```python
from build123d import *

# Parameters (mm, degrees)
ESQUISSE1_R             = 1.66
BOSS_EXTRU_1_DEPTH      = 2.5
ESQUISSE2_W             = 13.135596865
ESQUISSE2_H             = 97.305440857
ENL_V_MAT_EXTRU_1_DEPTH = 3.5


with BuildPart() as part:
    # Esquisse1 → Boss.-Extru.1 (new body)
    with BuildSketch(Plane.XY):
        with BuildLine():
            Line((-29.728572008, 42.160761401), (-21.428572008, 42.160761401))
            Line((-21.428572008, 42.160761401), (21.971427992, 42.160761401))
            Line((21.971427992, 42.160761401), (30.271427992, 42.160761401))
            Line((30.271427992, 42.160761401), (30.271427992, 36.160761401))
            ThreePointArc((30.271427992, 36.160761401), (25.904827727, 32.472835586), (24.271427992, 26.995610011))
            Line((24.271427992, 26.995610011), (24.271427992, -25.67408721))
            ThreePointArc((24.271427992, -25.67408721), (25.904827727, -31.151312785), (30.271427992, -34.839238599))
            Line((30.271427992, -34.839238599), (30.271427992, -40.839238599))
            Line((30.271427992, -40.839238599), (21.971427992, -40.839238599))
            Line((21.971427992, -40.839238599), (-21.428572008, -40.839238599))
            Line((-21.428572008, -40.839238599), (-29.728572008, -40.839238599))
            Line((-29.728572008, -40.839238599), (-29.728572008, -34.839238599))
            ThreePointArc((-29.728572008, -34.839238599), (-25.361971742, -31.151312785), (-23.728572008, -25.67408721))
            Line((-23.728572008, -25.67408721), (-23.728572008, 26.995610011))
            ThreePointArc((-23.728572008, 26.995610011), (-25.361971742, 32.472835586), (-29.728572008, 36.160761401))
            Line((-29.728572008, 36.160761401), (-29.728572008, 42.160761401))
        make_face()
        with Locations((-25.578572008, 39.160761401)):
            Circle(ESQUISSE1_R, mode=Mode.SUBTRACT)
        with Locations((26.121427992, 39.160761401)):
            Circle(ESQUISSE1_R, mode=Mode.SUBTRACT)
        with Locations((-25.578572008, -37.839238599)):
            Circle(ESQUISSE1_R, mode=Mode.SUBTRACT)
        with Locations((26.121427992, -37.839238599)):
            Circle(ESQUISSE1_R, mode=Mode.SUBTRACT)
        with BuildLine():
            Line((-9.728572008, 30.929161254), (10.271427992, 30.929161254))
            ThreePointArc((10.271427992, 30.929161254), (13.806961898, 29.46469516), (15.271427992, 25.929161254))
            Line((15.271427992, 25.929161254), (15.271427992, -24.607638453))
            ThreePointArc((15.271427992, -24.607638453), (13.806961898, -28.143172359), (10.271427992, -29.607638453))
            Line((10.271427992, -29.607638453), (-9.728572008, -29.607638453))
            ThreePointArc((-9.728572008, -29.607638453), (-13.264105914, -28.143172359), (-14.728572008, -24.607638453))
            Line((-14.728572008, -24.607638453), (-14.728572008, 25.929161254))
            ThreePointArc((-14.728572008, 25.929161254), (-13.264105914, 29.46469516), (-9.728572008, 30.929161254))
        make_face(mode=Mode.SUBTRACT)
    extrude(amount=BOSS_EXTRU_1_DEPTH)

    # Esquisse2 → Enlèv. mat.-Extru.1 (cut, through all)
    with BuildSketch(Plane(origin=(0, 0, 0), x_dir=(-1, 0, 0), z_dir=(0, 0, -1))):
        with Locations((-35.339226425, 0.262800476)):
            Rectangle(ESQUISSE2_W, ESQUISSE2_H)
        with Locations((34.79637044, 0.262800476)):
            Rectangle(ESQUISSE2_W, ESQUISSE2_H)
    extrude(amount=-ENL_V_MAT_EXTRU_1_DEPTH, mode=Mode.SUBTRACT)


solid = part.part
```
Work out the finished part from the listing and answer in its coordinate system (mm). A direction names the side the tool comes from. Give positions to 0.01 mm unless a question says otherwise; leave off trailing zeros. Loops run counter-clockwise (first coordinate to the right, second up) from the corner with the lowest first, then second, coordinate; pieces in that order, holes last. Notation, with made-up numbers: (50, -20) -> (77, -20) arc R13 cw to (77, 0) -> close; hole circle Ø6 at (16.25, 33). An arc over 180 degrees is marked (long way). Write item = value, one per line. Start each with the question number.
(1) The mould has two halves that part along Y. Classify faces 4 (the flat face through (-14.729, 0, 1)), 5 (the flat face through (-28.229, -37, 1)), 6 (the flat face through (0, 42.161, 1)): +Y half, -Y half, draft (parallel to the pull), parting line (faces both ways), or undercut.
(2) Find section C-C on z = 1.4. Give the vertices of the cut face in (x, y), and give its area (3 significant figures).
(3) Given pin 1 Ø2.5 at (x, y) = (26.12, 39.16) entering from -Z; pin 2 Ø1.5 at (y, z) = (-26, 1.5) entering from +X, each flat-ended and moving along its own axis, determine where each tip first touches the part or whether it passes through.
(4) Which of the six approach directions +Z, -Z, +X, -X, +Y, -Y give full straight-line access (tool end or side, diameter ignored) to faces 1 (the cylindrical face through (-24.893, 31.678, 1.232)), 2 (the flat face through (24.271, 1, 1)), 3 (the cylindrical face through (13.85, -28.1, 1.23))?
(5) Find section B-B on x = 5. Give the vertices of the cut face in (y, z).
(6) Find the intervals of material crossed by probe 1 along Y at (x, z) = (0, 1.1); probe 2 along X at (y, z) = (-11.5, 1.85); probe 3 along X at (y, z) = (-36.5, 1.5), in increasing order. Write a range as from..to.
(7) Find section A-A on y = 3. Give the vertices of the cut face in (x, z), and give its area (3 significant figures).
From the geometry:
q1.face_4 = undercut
q1.face_5 = draft
q1.face_6 = +Y half
q2.outline = (-28.23, -40.84) -> (28.77, -40.84) -> (28.77, -34.03) arc R10 cw to (24.27, -25.67) -> (24.27, 27) arc R10 cw to (28.77, 35.35) -> (28.77, 42.16) -> (-28.23, 42.16) -> (-28.23, 35.35) arc R10 cw to (-23.73, 27) -> (-23.73, -25.67) arc R10 cw to (-28.23, -34.03) -> close; hole circle Ø3.32 at (-25.58, -37.84); hole circle Ø3.32 at (-25.58, 39.16); hole (-14.73, -24.61) arc R5 ccw to (-9.73, -29.61) -> (10.27, -29.61) arc R5 ccw to (15.27, -24.61) -> (15.27, 25.93) arc R5 ccw to (10.27, 30.93) -> (-9.73, 30.93) arc R5 ccw to (-14.73, 25.93) -> close; hole circle Ø3.32 at (26.12, -37.84); hole circle Ø3.32 at (26.12, 39.16)
q2.area = 2,320 mm^2
q3.pin_1 = through
q3.pin_2 = 24.33
q4.face_1 = +Z, -Z, -X
q4.face_2 = +Z, -Z, +X
q4.face_3 = +Z, -Z
q5.outline = (-40.84, 0) -> (-29.61, 0) -> (-29.61, 2.5) -> (-40.84, 2.5) -> close; (30.93, 0) -> (42.16, 0) -> (42.16, 2.5) -> (30.93, 2.5) -> close
q6.probe_1 = -40.84..-29.61, 30.93..42.16
q6.probe_2 = -23.73..-14.73, 15.27..24.27
q6.probe_3 = -28.23..-26.56, -24.6..25.14, 27.1..28.77
q7.outline = (-23.73, 0) -> (-14.73, 0) -> (-14.73, 2.5) -> (-23.73, 2.5) -> close; (15.27, 0) -> (24.27, 0) -> (24.27, 2.5) -> (15.27, 2.5) -> close
q7.area = 45.0 mm^2
